Check sheet for the modelled part. Datum: model origin and axes. Units: mm. A direction names the side the tool comes from. Round coordinates to 2 decimals unless told otherwise and drop trailing zeros. Order: outer loops, then holes, each group sorted by start corner. A loop starts at its lowest first (then second) coordinate and runs counter-clockwise, first axis right, second up. Notation, with made-up numbers: (37.5, 26.5) -> (82.5, 26.5) arc R7 ccw to (82.5, 35.5) -> close; hole circle Ø9 at (-12.75, 51). An arc over 180 degrees is marked (long way). Answer in a Markdown table with one row per item.
Autodesk Inventor part; units mm, degrees
ref_plane "YZ Plane" through (0, 0, 0) normal (1, 0, 0) x (0, 1, 0)
ref_plane "XZ Plane" through (0, 0, 0) normal (0, 1, 0) x (-1, 0, 0)
ref_plane "XY Plane" through (0, 0, 0) normal (0, 0, 1) x (1, 0, 0)
sketch "スケッチ1" plane through (0, 0, 0) normal (0, 0, 1) x (1, 0, 0)
  circle A0 centre (0, 0) radius 13.75
  line L0 (0, 13.75) -> (0, -13.75) construction
  line L1 (13.75, 0) -> (-13.75, 0) construction
  circle A1 centre (0, 0) radius 5
  point P0 (0, 8.75)
  point P1 (0, -8.75)
  point P2 (8.75, 0)
  point P3 (-8.75, 0)
  dimension "d0" = 27.5
  dimension "d1" = 17.5
  dimension "d2" = 17.5
  dimension "d3" = 10
extrude "押し出し1" add sketch "スケッチ1" along normal blind 2 contours A0 | A1
extrude "押し出し2" add sketch "スケッチ1" against normal blind 4.7 contours A1
hole "穴1" at (0, 0, 0) at (0, 8.75, 0) at (0, -8.75, 0) at (8.75, 0, 0) at (-8.75, 0, 0) direction (0, 0, -1) diameter 3.2 depth 8 tip angle 118
hole "穴2" at (-8.75, 0, 0) at (0, 8.75, 0) at (8.75, 0, 0) at (0, -8.75, 0) at (0, 0, 0) direction (0, 0, 1) diameter 3.2 depth 8 tip angle 118
sketch "スケッチ3" plane through (0, 0, 2) normal (0, 0, 1) x (1, 0, 0)
  circle A0 centre (0, -8.75) radius 1.6
  circle A1 centre (0, 8.75) radius 1.6
  circle A2 centre (-8.75, 0) radius 1.6
  circle A3 centre (8.75, 0) radius 1.6
  circle A4 centre (0, 0) radius 1.6
  circle A5 centre (0, 0) radius 13.75
properties part number "servo horn wide"
Item 1: Cross-section at A-A (x = 0). Record the boundary of the cut face in (y, z).
Result sheet:
| item | result |
|---|---|
| outline | (-13.75, 0) -> (-10.35, 0) -> (-10.35, 2) -> (-13.75, 2) -> close; (-7.15, 0) -> (-5, 0) -> (-5, -4.7) -> (-1.6, -4.7) -> (-1.6, 2) -> (-7.15, 2) -> close; (1.6, -4.7) -> (5, -4.7) -> (5, 0) -> (7.15, 0) -> (7.15, 2) -> (1.6, 2) -> close; (10.35, 0) -> (13.75, 0) -> (13.75, 2) -> (10.35, 2) -> close |
Item 2: Cross-section at C-C (x = -8.75). Record the boundary of the cut face in (y, z), and give its area (3 significant figures).
Result sheet:
| item | result |
|---|---|
| outline | (-10.61, 0) -> (-1.6, 0) -> (-1.6, 2) -> (-10.61, 2) -> close; (1.6, 0) -> (10.61, 0) -> (10.61, 2) -> (1.6, 2) -> close |
| area | 36.0 mm^2 |
Item 3: Scan lines: line 1 (Y direction, x = 0, z = 1.5); line 2 (Z direction, x = 8.75, y = -7.5); line 3 (Y direction, x = 9.5, z = 0.75). Record each from-to range of solid material in increasing order. Write a range as [from, to].
Result sheet:
| item | result |
|---|---|
| line 1 | y = [-13.75, -10.35], [-7.15, -1.6], [1.6, 7.15], [10.35, 13.75] |
| line 2 | z = [0, 2] |
| line 3 | y = [-9.94, -1.41], [1.41, 9.94] |
Item 4: Cross-section at B-B (y = 8.5). Record the boundary of the cut face in (x, z), and give its area (3 significant figures).
Result sheet:
| item | result |
|---|---|
| outline | (-10.81, 0) -> (-1.58, 0) -> (-1.58, 2) -> (-10.81, 2) -> close; (1.58, 0) -> (10.81, 0) -> (10.81, 2) -> (1.58, 2) -> close |
| area | 36.9 mm^2 |
Item 5: Depth check by flat-ended pin: P1, Ø1, axis at x = -8, y = 1, coming from the -Z side. Enter the tip coordinate at first touch or a pass-through.
Result sheet:
| item | result |
|---|---|
| P1 | stops at z = 0 |
Item 6: Set-up check for faces 1 (the cylindrical face through (-0.07, -10.35, 1.01)), 2 (the flat face through (0, -6, 0)): record each of +Z, -Z, +X, -X, +Y, -Y from which the full face is reachable in a straight line by a thin tool's end or side.
Result sheet:
| item | result |
|---|---|
| face 1 | +Z, -Z |
| face 2 | -Z |
Item 7: Mould release check, pull along X, two halves, no side actions. Record for faces 3 (the flat face through (2, 0, -4.7)), 4 (the cylindrical face through (-1.08, -4.88, -2.32)), 5 (the cylindrical face through (10.31, -0.35, 1.01)): pulls with the +X half, pulls with the -X half, needs draft (parallel to the pull), parting line crosses it, or undercut.
Result sheet:
| item | result |
|---|---|
| face 3 | needs draft |
| face 4 | parting line crosses it |
| face 5 | undercut |
Item 8: Cross-section at D-D (z = 1). Record the boundary of the cut face in (x, y).
Result sheet:
| item | result |
|---|---|
| outline | circle Ø27.5 at (0, 0); hole circle Ø3.2 at (-8.75, 0); hole circle Ø3.2 at (0, -8.75); hole circle Ø3.2 at (0, 0); hole circle Ø3.2 at (0, 8.75); hole circle Ø3.2 at (8.75, 0) |
